Source: CAD feature listing. Evaluate the final solid. Frame: model axes, mm. A direction names the side the tool comes from. Round coordinates to 2 decimals unless told otherwise and drop trailing zeros. Order: outer loops, then holes, each group sorted by start corner. A loop starts at its lowest first (then second) coordinate and runs counter-clockwise, first axis right, second up. Notation, with made-up numbers: M 83.5,68.5 L 138.5,68.5 A5 cw 138.5,72.5 Z; hole C 63.25,43 d10. An arc over 180 degrees is marked long. Use one line per item in the form item = value. Start each with the question number.
Q1. Section C-C (x = 15). Return the cut outline in (y, z), plus the area to 3 significant figures.
Q2. Section B-B (y = 2). Return the cut outline in (x, z).
Q3. Section A-A (z = 0). Return the cut outline in (x, y), plus the area to 3 significant figures.
Q4. Reachability of faces 4 (the cylindrical face through (13.476, 2.712, 0.632)), 5 (the cylindrical face through (-0.65, 5.07, 1.01)), 6 (the flat face through (0, 20, 0)) from +Z, -Z, +X, -X, +Y, -Y: full face, straight path, thin tool, end or side. Return the list, or none.
Q5. Section D-D (x = -15). Return the cut outline in (y, z), plus the area to 3 significant figures.
Q6. Pull-direction query (Y, two-part tool) for faces 1 (the cylindrical face through (0.215, 2.712, 13.364)), 2 (the flat face through (0, 0, 4)), 3 (the cylindrical face through (12.58, 16.11, -0.46)); classes: pulls with the +Y half, pulls with the -Y half, needs draft (parallel to the pull), parting line crosses it, or undercut.
Q7. Material intervals for probe 1 along Z at (x, y) = (0, 1.5); probe 2 along Z at (x, y) = (0, -6); probe 3 along X at (y, z) = (0.5, -1.5), sorted ascending.
Q8. Contact query for flat-ended pins moving along their axis: pin 1 (12 mm diameter, centred on x = -9.5, z = 9, fed in from -Y); pin 2 (1 mm diameter, centred on y = 13.5, z = -7, fed in from +X); pin 3 (3 mm diameter, centred on x = -15, z = 0, fed in from -Y). Output: stop coordinate, or through.
from build123d import *

# Parameters (mm, degrees)
SKETCH1_R           = 19.95
BOSS_EXTRUDE1_DEPTH = 20
SKETCH6_R           = 1.2
SKETCH12_R          = 1.9
BOSS_EXTRUDE2_DEPTH = 10
SKETCH13_R          = 0.9
CUT_EXTRUDE1_DEPTH  = 10
SKETCH14_R          = 1.65
CUT_EXTRUDE2_DEPTH  = 5.5


with BuildPart() as part:
    # Sketch1 → Boss-Extrude1 (new body)
    with BuildSketch(Plane(origin=(0, 0, 0), x_dir=(1, 0, 0), z_dir=(0, 1, 0))):
        Circle(SKETCH1_R)
    extrude(amount=BOSS_EXTRUDE1_DEPTH)

    # Cut-Sweep2: sweep along a path in Sketch5
    with BuildLine(Plane.XY) as cut_sweep2_path:
        Line((0, 0), (0, 10))
        ThreePointArc((0, 10), (1.464466094, 13.535533906), (5, 15))
        Line((5, 15), (19.95, 15))
    # Sketch6 → Cut-Sweep2 (sweep, cut)
    with BuildSketch(Plane(origin=(0, 0, 0), x_dir=(-1, 0, 0), z_dir=(0, -1, 0))):
        Circle(SKETCH6_R)
    sweep(path=cut_sweep2_path.line, mode=Mode.SUBTRACT)

    # Sketch12 → Boss-Extrude2 (add)
    with BuildSketch(Plane(origin=(0, 0, 0), x_dir=(-1, 0, 0), z_dir=(0, -1, 0))):
        Circle(SKETCH12_R)
    extrude(amount=BOSS_EXTRUDE2_DEPTH)

    # Sketch13 → Cut-Extrude1 (cut)
    with BuildSketch(Plane(origin=(0, -10, 0), x_dir=(-1, 0, 0), z_dir=(0, -1, 0))):
        Circle(SKETCH13_R)
    extrude(amount=-CUT_EXTRUDE1_DEPTH, mode=Mode.SUBTRACT)

    # Sketch14 → Cut-Extrude2 (cut)
    with BuildSketch(Plane(origin=(0, 0, 0), x_dir=(-1, 0, 0), z_dir=(0, -1, 0))):
        with Locations((-15, 0)):
            Circle(SKETCH14_R)
        with Locations((0, 15)):
            Circle(SKETCH14_R)
        with Locations((0, -15)):
            Circle(SKETCH14_R)
        with Locations((15, 0)):
            Circle(SKETCH14_R)
    extrude(amount=-CUT_EXTRUDE2_DEPTH, mode=Mode.SUBTRACT)


solid = part.part
Results list:
q1.outline = M 0,-13.15 L 20,-13.15 L 20,13.15 L 0,13.15 L 0,1.65 L 5.5,1.65 L 5.5,-1.65 L 0,-1.65 Z; hole C 15,0 d2.4
q1.area = 503 mm2
q2.outline = C 0,0 d39.9; hole C -15,0 d3.3; hole C 0,-15 d3.3; hole C 0,15 d3.3; hole C 0,0 d2.4; hole C 15,0 d3.3
q3.outline = M -19.95,0 L -16.65,0 L -16.65,5.5 L -13.35,5.5 L -13.35,0 L -1.9,0 L -1.9,-10 L -0.9,-10 L -0.9,0 L -1.2,0 L -1.2,10 A6.2 cw 5,16.2 L 19.95,16.2 L 19.95,20 L -19.95,20 Z; M 0.9,-10 L 1.9,-10 L 1.9,0 L 13.35,0 L 13.35,5.5 L 16.65,5.5 L 16.65,0 L 19.95,0 L 19.95,13.8 L 5,13.8 A3.8 ccw 1.2,10 L 1.2,0 L 0.9,0 Z
q3.area = 703 mm2
q4.face_4 = -Y
q4.face_5 = none
q4.face_6 = +Z, -Z, +X, -X, +Y
q5.outline = M 0,-13.15 L 20,-13.15 L 20,13.15 L 0,13.15 L 0,1.65 L 5.5,1.65 L 5.5,-1.65 L 0,-1.65 Z
q5.area = 508 mm2
q6.face_1 = needs draft
q6.face_2 = pulls with the -Y half
q6.face_3 = undercut
q7.probe_1 = -19.95 to -16.65, -13.35 to -1.2, 1.2 to 13.35, 16.65 to 19.95
q7.probe_2 = -1.9 to -0.9, 0.9 to 1.9
q7.probe_3 = -19.89 to -15.69, -14.31 to 14.31, 15.69 to 19.89
q8.pin_1 = 0
q8.pin_2 = 18.86
q8.pin_3 = 5.5
